```python
from build123d import *

# Parameters (mm, degrees)
SKETCH1_W           = 113
SKETCH1_H           = 130
BOSS_EXTRUDE1_DEPTH = 5
FILLET1_R           = 2
SKETCH3_W           = 75
SKETCH3_H           = 28
CUT_EXTRUDE1_DEPTH  = 4


with BuildPart() as part:
    # Sketch1 → Boss-Extrude1 (new body)
    with BuildSketch(Plane(origin=(0, 0, 0), x_dir=(1, 0, 0), z_dir=(0, 1, 0))):
        Rectangle(SKETCH1_W, SKETCH1_H)
    extrude(amount=BOSS_EXTRUDE1_DEPTH)

    # Fillet1
    fillet1_edges = [part.edges().sort_by_distance(p)[0] for p in [
        (56.5, 2.5, 65),
        (-56.5, 2.5, 65),
        (-56.5, 2.5, -65),
        (56.5, 2.5, -65),
    ]]
    fillet(fillet1_edges, radius=FILLET1_R)

    # Sketch3 → Cut-Extrude1 (cut)
    with BuildSketch(Plane(origin=(0, 5, 0), x_dir=(1, 0, 0), z_dir=(0, 1, 0))):
        with Locations((0, 29.689320388)):
            Rectangle(SKETCH3_W, SKETCH3_H)
    extrude(amount=-CUT_EXTRUDE1_DEPTH, mode=Mode.SUBTRACT)


solid = part.part
```
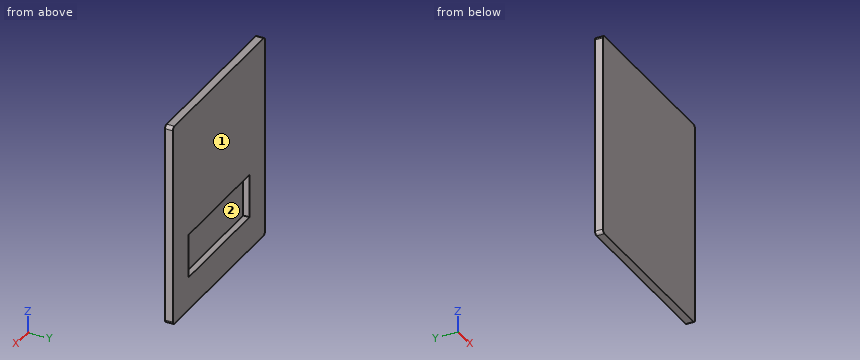
Verification items for the finished model (mm, model axes). Face numbers are marked on the shaded views. Round coordinates to 2 decimals unless told otherwise and drop trailing zeros. Write each loop counter-clockwise with the first axis right and the second up, starting at its lowest first coordinate (ties: lowest second). Pieces come first, ordered by that corner, then holes. Notation, with made-up numbers: (10, 79) -> (21, 79) arc R23 ccw to (21, 115) -> close; hole circle Ø10 at (14.5, -27). An arc over 180 degrees is marked (long way). Write each question's results on one line, items separated by ' | '. Start each with the question number.
1. Draft check along X on the marked faces 1 and 2. Enter one of: +X half, -X half, draft (parallel to the pull), parting line (faces both ways), or undercut.
2. Cross-section at B-B (x = -12). Enter the section's corners in (y, z), then the cut area to 3 significant figures.
3. Cross-section at A-A (y = 3.05). Enter the section's corners in (x, z).
4. Material ranges on probe 1 along X at (y, z) = (2.9, -21.5); probe 2 along Z at (x, y) = (6.5, 3.3); probe 3 along Y at (x, z) = (-19, -16), recorded low to high. Write a range as from..to.
Solutions:
1) face 1: draft | face 2: undercut
2) outline: (0, -65) -> (5, -65) -> (5, -43.69) -> (1, -43.69) -> (1, -15.69) -> (5, -15.69) -> (5, 65) -> (0, 65) -> close | area: 538 mm2
3) outline: (-56.5, -63) arc R2 ccw to (-54.5, -65) -> (54.5, -65) arc R2 ccw to (56.5, -63) -> (56.5, 63) arc R2 ccw to (54.5, 65) -> (-54.5, 65) arc R2 ccw to (-56.5, 63) -> close; hole (-37.5, -43.69) -> (37.5, -43.69) -> (37.5, -15.69) -> (-37.5, -15.69) -> close
4) probe 1: x = -56.5..-37.5, 37.5..56.5 | probe 2: z = -65..-43.69, -15.69..65 | probe 3: y = 0..1
